Part model, mm, in its own coordinate system. Give positions to 0.01 mm unless a question says otherwise; leave off trailing zeros. Write each loop counter-clockwise with the first axis right and the second up, starting at its lowest first coordinate (ties: lowest second). Pieces come first, ordered by that corner, then holes.
```python
from build123d import *

# Parameters (mm, degrees)
CROQUIS1_W                = 38.1
CROQUIS1_H                = 38.1
SALIENTE_EXTRUIR1_DEPTH   = 80
SALIENTE_EXTRUIR1_2_DEPTH = 80
SALIENTE_EXTRUIR1_3_DEPTH = 80
SALIENTE_EXTRUIR1_4_DEPTH = 80
SALIENTE_EXTRUIR1_5_DEPTH = 80
SALIENTE_EXTRUIR1_6_DEPTH = 80
CROQUIS2_W                = 1894.3
CROQUIS2_H                = 676.2
SALIENTE_EXTRUIR2_DEPTH   = 25.4
CROQUIS3_W                = 38.1
CROQUIS3_H                = 38.1
SALIENTE_EXTRUIR3_DEPTH   = 450
CROQUIS4_W                = 1894.3
CROQUIS4_H                = 676.2
SALIENTE_EXTRUIR4_DEPTH   = 25.4
CROQUIS5_W                = 38.1
CROQUIS5_H                = 38.1
SALIENTE_EXTRUIR5_DEPTH   = 450
CROQUIS6_W                = 1894.3
CROQUIS6_H                = 676.2
SALIENTE_EXTRUIR6_DEPTH   = 25.4
CROQUIS7_W                = 38.1
CROQUIS7_H                = 38.1
SALIENTE_EXTRUIR7_DEPTH   = 450
CROQUIS8_W                = 1894.3
CROQUIS8_H                = 676.2
SALIENTE_EXTRUIR8_DEPTH   = 25.4
CROQUIS9_W                = 38.1
CROQUIS9_H                = 38.1
SALIENTE_EXTRUIR9_DEPTH   = 450
CROQUIS10_W               = 1894.3
CROQUIS10_H               = 676.2
SALIENTE_EXTRUIR10_DEPTH  = 25.4


with BuildPart() as part:
    # Croquis1 → Saliente-Extruir1 (new body)
    with BuildSketch(Plane(origin=(0, 0, 0), x_dir=(1, 0, 0), z_dir=(0, 1, 0))):
        with Locations((19.05, -19.05)):
            Rectangle(CROQUIS1_W, CROQUIS1_H)
    extrude(amount=SALIENTE_EXTRUIR1_DEPTH)



with BuildPart() as body_2:
    # Croquis1 → Saliente-Extruir1 2 (new body)
    with BuildSketch(Plane(origin=(0, 0, 0), x_dir=(1, 0, 0), z_dir=(0, 1, 0))):
        with Locations((947.15, -19.05)):
            Rectangle(CROQUIS1_W, CROQUIS1_H)
    extrude(amount=SALIENTE_EXTRUIR1_2_DEPTH)


with BuildPart() as body_3:
    # Croquis1 → Saliente-Extruir1 3 (new body)
    with BuildSketch(Plane(origin=(0, 0, 0), x_dir=(1, 0, 0), z_dir=(0, 1, 0))):
        with Locations((1875.25, -19.05)):
            Rectangle(CROQUIS1_W, CROQUIS1_H)
    extrude(amount=SALIENTE_EXTRUIR1_3_DEPTH)


with BuildPart() as body_4:
    # Croquis1 → Saliente-Extruir1 4 (new body)
    with BuildSketch(Plane(origin=(0, 0, 0), x_dir=(1, 0, 0), z_dir=(0, 1, 0))):
        with Locations((1875.25, -657.15)):
            Rectangle(CROQUIS1_W, CROQUIS1_H)
    extrude(amount=SALIENTE_EXTRUIR1_4_DEPTH)


with BuildPart() as body_5:
    # Croquis1 → Saliente-Extruir1 5 (new body)
    with BuildSketch(Plane(origin=(0, 0, 0), x_dir=(1, 0, 0), z_dir=(0, 1, 0))):
        with Locations((947.15, -657.15)):
            Rectangle(CROQUIS1_W, CROQUIS1_H)
    extrude(amount=SALIENTE_EXTRUIR1_5_DEPTH)


with BuildPart() as body_6:
    # Croquis1 → Saliente-Extruir1 6 (new body)
    with BuildSketch(Plane(origin=(0, 0, 0), x_dir=(1, 0, 0), z_dir=(0, 1, 0))):
        with Locations((19.05, -657.15)):
            Rectangle(CROQUIS1_W, CROQUIS1_H)
    extrude(amount=SALIENTE_EXTRUIR1_6_DEPTH)


with BuildPart() as part_1:
    add(part.part)

    add(body_2.part)  # Saliente-Extruir2 merges body 2

    add(body_3.part)  # Saliente-Extruir2 merges body 3

    add(body_4.part)  # Saliente-Extruir2 merges body 4

    add(body_5.part)  # Saliente-Extruir2 merges body 5

    add(body_6.part)  # Saliente-Extruir2 merges body 6
    # Croquis2 → Saliente-Extruir2 (add)
    with BuildSketch(Plane(origin=(0, 80, 0), x_dir=(1, 0, 0), z_dir=(0, 1, 0))):
        with Locations((947.15, -338.1)):
            Rectangle(CROQUIS2_W, CROQUIS2_H)
    extrude(amount=SALIENTE_EXTRUIR2_DEPTH)

    # Croquis3 → Saliente-Extruir3 (add)
    with BuildSketch(Plane(origin=(0, 105.4, 0), x_dir=(1, 0, 0), z_dir=(0, 1, 0))):
        with Locations((19.05, -19.05)):
            Rectangle(CROQUIS3_W, CROQUIS3_H)
        with Locations((947.15, -19.05)):
            Rectangle(CROQUIS3_W, CROQUIS3_H)
        with Locations((1875.25, -19.05)):
            Rectangle(CROQUIS3_W, CROQUIS3_H)
        with Locations((1875.25, -657.15)):
            Rectangle(CROQUIS3_W, CROQUIS3_H)
        with Locations((947.15, -657.15)):
            Rectangle(CROQUIS3_W, CROQUIS3_H)
        with Locations((19.05, -657.15)):
            Rectangle(CROQUIS3_W, CROQUIS3_H)
    extrude(amount=SALIENTE_EXTRUIR3_DEPTH)

    # Croquis4 → Saliente-Extruir4 (add)
    with BuildSketch(Plane(origin=(0, 555.4, 0), x_dir=(1, 0, 0), z_dir=(0, 1, 0))):
        with Locations((947.15, -338.1)):
            Rectangle(CROQUIS4_W, CROQUIS4_H)
    extrude(amount=SALIENTE_EXTRUIR4_DEPTH)

    # Croquis5 → Saliente-Extruir5 (add)
    with BuildSketch(Plane(origin=(0, 580.8, 0), x_dir=(1, 0, 0), z_dir=(0, 1, 0))):
        with Locations((19.05, -19.05)):
            Rectangle(CROQUIS5_W, CROQUIS5_H)
        with Locations((947.15, -19.05)):
            Rectangle(CROQUIS5_W, CROQUIS5_H)
        with Locations((1875.25, -19.05)):
            Rectangle(CROQUIS5_W, CROQUIS5_H)
        with Locations((1875.25, -657.15)):
            Rectangle(CROQUIS5_W, CROQUIS5_H)
        with Locations((947.15, -657.15)):
            Rectangle(CROQUIS5_W, CROQUIS5_H)
        with Locations((19.05, -657.15)):
            Rectangle(CROQUIS5_W, CROQUIS5_H)
    extrude(amount=SALIENTE_EXTRUIR5_DEPTH)

    # Croquis6 → Saliente-Extruir6 (add)
    with BuildSketch(Plane(origin=(0, 1030.8, 0), x_dir=(1, 0, 0), z_dir=(0, 1, 0))):
        with Locations((947.15, -338.1)):
            Rectangle(CROQUIS6_W, CROQUIS6_H)
    extrude(amount=SALIENTE_EXTRUIR6_DEPTH)

    # Croquis7 → Saliente-Extruir7 (add)
    with BuildSketch(Plane(origin=(0, 1056.2, 0), x_dir=(1, 0, 0), z_dir=(0, 1, 0))):
        with Locations((19.05, -19.05)):
            Rectangle(CROQUIS7_W, CROQUIS7_H)
        with Locations((947.15, -19.05)):
            Rectangle(CROQUIS7_W, CROQUIS7_H)
        with Locations((1875.25, -19.05)):
            Rectangle(CROQUIS7_W, CROQUIS7_H)
        with Locations((1875.25, -657.15)):
            Rectangle(CROQUIS7_W, CROQUIS7_H)
        with Locations((947.15, -657.15)):
            Rectangle(CROQUIS7_W, CROQUIS7_H)
        with Locations((19.05, -657.15)):
            Rectangle(CROQUIS7_W, CROQUIS7_H)
    extrude(amount=SALIENTE_EXTRUIR7_DEPTH)

    # Croquis8 → Saliente-Extruir8 (add)
    with BuildSketch(Plane(origin=(0, 1506.2, 0), x_dir=(1, 0, 0), z_dir=(0, 1, 0))):
        with Locations((947.15, -338.1)):
            Rectangle(CROQUIS8_W, CROQUIS8_H)
    extrude(amount=SALIENTE_EXTRUIR8_DEPTH)

    # Croquis9 → Saliente-Extruir9 (add)
    with BuildSketch(Plane(origin=(0, 1531.6, 0), x_dir=(1, 0, 0), z_dir=(0, 1, 0))):
        with Locations((19.05, -19.05)):
            Rectangle(CROQUIS9_W, CROQUIS9_H)
        with Locations((947.15, -19.05)):
            Rectangle(CROQUIS9_W, CROQUIS9_H)
        with Locations((1875.25, -19.05)):
            Rectangle(CROQUIS9_W, CROQUIS9_H)
        with Locations((1875.25, -657.15)):
            Rectangle(CROQUIS9_W, CROQUIS9_H)
        with Locations((947.15, -657.15)):
            Rectangle(CROQUIS9_W, CROQUIS9_H)
        with Locations((19.05, -657.15)):
            Rectangle(CROQUIS9_W, CROQUIS9_H)
    extrude(amount=SALIENTE_EXTRUIR9_DEPTH)

    # Croquis10 → Saliente-Extruir10 (add)
    with BuildSketch(Plane(origin=(0, 1981.6, 0), x_dir=(1, 0, 0), z_dir=(0, 1, 0))):
        with Locations((947.15, -338.1)):
            Rectangle(CROQUIS10_W, CROQUIS10_H)
    extrude(amount=SALIENTE_EXTRUIR10_DEPTH)


solid = part_1.part
```
1) Two-plate mould, pull along Y, no slides. Class faces 1 (the face through (934, 1030.8, 333)), 2 (the face through (0, 1147, 640)), 3 (the face through (934, 2007, 333)), 4 (the face through (934, 555.4, 333)): +Y half, -Y half, draft (parallel to the pull), parting line (faces both ways), or undercut.
Answers follow:
face 1: undercut
face 2: draft
face 3: +Y half
face 4: undercut
2) Saw through at C-C, the plane z = 284. Write the cut outline in (x, y), then the cut area to 3 significant figures.
Answers follow:
outline: (0, 80) - (1894.3, 80) - (1894.3, 105.4) - (0, 105.4) - close; (0, 555.4) - (1894.3, 555.4) - (1894.3, 580.8) - (0, 580.8) - close; (0, 1030.8) - (1894.3, 1030.8) - (1894.3, 1056.2) - (0, 1056.2) - close; (0, 1506.2) - (1894.3, 1506.2) - (1894.3, 1531.6) - (0, 1531.6) - close; (0, 1981.6) - (1894.3, 1981.6) - (1894.3, 2007) - (0, 2007) - close
area: 241,000 mm2
3) Saw through at A-A, the plane x = 1117. Write the cut outline in (y, z).
Answers follow:
outline: (80, 0) - (105.4, 0) - (105.4, 676.2) - (80, 676.2) - close; (555.4, 0) - (580.8, 0) - (580.8, 676.2) - (555.4, 676.2) - close; (1030.8, 0) - (1056.2, 0) - (1056.2, 676.2) - (1030.8, 676.2) - close; (1506.2, 0) - (1531.6, 0) - (1531.6, 676.2) - (1506.2, 676.2) - close; (1981.6, 0) - (2007, 0) - (2007, 676.2) - (1981.6, 676.2) - close
4) Saw through at B-B, the plane y = 615. Write the cut outline in (x, z), then the cut area to 3 significant figures.
Answers follow:
outline: (0, 0) - (38.1, 0) - (38.1, 38.1) - (0, 38.1) - close; (0, 638.1) - (38.1, 638.1) - (38.1, 676.2) - (0, 676.2) - close; (928.1, 0) - (966.2, 0) - (966.2, 38.1) - (928.1, 38.1) - close; (928.1, 638.1) - (966.2, 638.1) - (966.2, 676.2) - (928.1, 676.2) - close; (1856.2, 0) - (1894.3, 0) - (1894.3, 38.1) - (1856.2, 38.1) - close; (1856.2, 638.1) - (1894.3, 638.1) - (1894.3, 676.2) - (1856.2, 676.2) - close
area: 8,710 mm2
5) Wall check: L1, parallel to Y at x = 304, z = 343; L2, parallel to Z at x = 948, y = 621.5. Give the ranges that are in metal, low to high.
Answers follow:
L1: y = 80 to 105.4, 555.4 to 580.8, 1030.8 to 1056.2, 1506.2 to 1531.6, 1981.6 to 2007
L2: z = 0 to 38.1, 638.1 to 676.2
